from build123d import *

# Parameters (mm, degrees)
EXTRUDE1_DEPTH = 82.55
SKETCH8_W      = 9.6647
SKETCH8_H      = 25.4
EXTRUDE6_DEPTH = 27.94
FILLET1_R      = 3.81


with BuildPart() as part:
    # Sketch1 → Extrude1 (new body)
    with BuildSketch(Plane.XY):
        Polygon((0, 0), (30.48, 0), (30.48, -5.08), (17.717260633, -5.08), (20.6502, -10.16), (6.35, -10.16), (6.35, -3.302), (-6.35, -3.302), (-6.35, -10.16), (-20.6502, -10.16), (-17.717260633, -5.08), (-30.48, -5.08), (-30.48, 0), align=None)
    extrude(amount=EXTRUDE1_DEPTH)

    # Sketch8 → Extrude6 (add)
    with BuildSketch(Plane(origin=(0, 0, 0), x_dir=(1, 0, 0), z_dir=(0, 1, 0))):
        with Locations((25.64765, -69.85)):
            Rectangle(SKETCH8_W, SKETCH8_H)
    extrude6 = extrude(amount=EXTRUDE6_DEPTH)

    # Fillet1
    fillet1_edges = [part.edges().sort_by_distance(p)[0] for p in [
        (30.48, -2.54, 0),
        (-30.48, -2.54, 0),
        (30.48, 11.43, 82.55),
        (-30.48, -2.54, 82.55),
    ]]
    fillet(fillet1_edges, radius=FILLET1_R)

    # Mirror1: Extrude6 across plane
    add(extrude6.mirror(Plane(origin=(0, 0, 0), x_dir=(0, 0, 1), z_dir=(1, 0, 0))))


solid = part.part
Can you work these out from the model? Positions are in its coordinate system, mm. A direction names the side the tool comes from. Give positions to 0.01 mm unless a question says otherwise; leave off trailing zeros. Loops run counter-clockwise (first coordinate to the right, second up) from the corner with the lowest first, then second, coordinate; pieces in that order, holes last. Notation, with made-up numbers: (-21.5, 68) - (-6.5, 68) arc R30 ccw to (-6.5, 98) - close; hole circle Ø7 at (14.25, 71.25). An arc over 180 degrees is marked (long way). Answer as a JSON object with one key per item and string values.
Q1. Imagine slicing it at C-C on z = 67. Write out the boundary of the cut face in (x, y), plus the area to 3 significant figures.
Geometry says:
{"outline": "(-30.48, -5.08) - (-17.72, -5.08) - (-20.65, -10.16) - (-6.35, -10.16) - (-6.35, -3.3) - (6.35, -3.3) - (6.35, -10.16) - (20.65, -10.16) - (17.72, -5.08) - (30.48, -5.08) - (30.48, 27.94) - (20.82, 27.94) - (20.82, 0) - (-20.82, 0) - (-20.82, 27.94) - (-30.48, 27.94) - close", "area": "958 mm²"}
Q2. Imagine slicing it at A-A on y = 1. Write out the boundary of the cut face in (x, z).
Geometry says:
{"outline": "(-30.48, 57.15) - (-20.82, 57.15) - (-20.82, 82.55) - (-30.48, 82.55) - close; (20.82, 57.15) - (30.48, 57.15) - (30.48, 78.74) arc R3.81 ccw to (26.67, 82.55) - (20.82, 82.55) - close"}
Q3. If we mould it in two halves opening along Y, with no side actions, what happens to faces 1 (the flat face through (-13, -10.16, 41)), 2 (the flat face through (6.35, -7, 41)), 3 (the flat face through (-24, -5.08, 41))? For each: pulls with the +Y half, pulls with the -Y half, needs draft (parallel to the pull), parting line crosses it, or undercut.
Geometry says:
{"face 1": "pulls with the -Y half", "face 2": "needs draft", "face 3": "undercut"}
Q4. Imagine slicing it at D-D on y = -7. Write out the boundary of the cut face in (x, z).
Geometry says:
{"outline": "(-18.83, 0) - (-6.35, 0) - (-6.35, 82.55) - (-18.83, 82.55) - close; (6.35, 0) - (18.83, 0) - (18.83, 82.55) - (6.35, 82.55) - close"}
Q5. Imagine slicing it at B-B on x = -22. Write out the boundary of the cut face in (y, z), plus the area to 3 significant figures.
Geometry says:
{"outline": "(-5.08, 0) - (0, 0) - (0, 57.15) - (27.94, 57.15) - (27.94, 82.55) - (-5.08, 82.55) - close", "area": "1,130 mm²"}
Q6. Which directions (+Z, -Z, +X, -X, +Y, -Y) give clear straight access to the entire face, cutting with the end or side of a thin tool? Please do faces 4 (the flat face through (24, -5.08, 41)), 5 (the flat face through (20.815, 14, 70)), 6 (the flat face through (-26, 14, 57.15)), 7 (the flat face through (0, -3.302, 41)).
Geometry says:
{"face 4": "+Z, -Z, +X", "face 5": "+Z, -Z, +Y", "face 6": "-Z, +X, -X, +Y", "face 7": "+Z, -Z, -Y"}
Q7. Will these pins go through, and if not, where does the flat tip stop? P1, Ø4, axis at x = 2.5, z = 23, coming from the -Y side; P2, Ø1.1, axis at x = -29.5, z = 81, coming from the -Y side; P3, Ø2, axis at y = -6.5, z = 49.5, coming from the +X side.
Geometry says:
{"P1": "y = -3.3", "P2": "y = -5.08", "P3": "x = 19.11"}
Q8. If I drill on L1, parallel to X at y = 11.5, z = 65; L2, parallel to Y at x = 3.5, z = 27; L3, parallel to Y at x = 16, z = 9.5, over which ranges is the centre line in solid material (lowest first)?
Geometry says:
{"L1": "-30.48 to -20.82, 20.82 to 30.48", "L2": "-3.3 to 0", "L3": "-10.16 to 0"}
